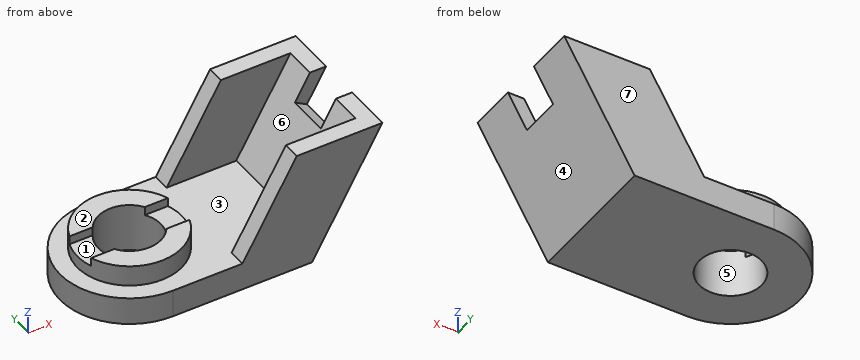
from build123d import *

# Parameters (mm, degrees)
F0_W      = 40
F0_H      = 8
F1_DEPTH  = 40
F3_DEPTH  = 8
F4_R      = 15
F5_DEPTH  = 6
F6_R      = 9
F7_DEPTH  = 14.001
F8_W      = 33.766868
F8_H      = 10
F9_DEPTH  = 2.5
F11_DEPTH = 40
F13_DEPTH = 5
F15_DEPTH = 5
F16_W     = 12
F16_H     = 11
F17_DEPTH = 5


with BuildPart() as f1:
    # F0 (on Front) → F1 (new body)
    with BuildSketch(Plane.XZ):
        with Locations((-20, -4)):
            Rectangle(F0_W, F0_H)
    extrude(amount=F1_DEPTH)

    # F2 (on face) → F3 (join)
    with BuildSketch(Plane.XY):
        with BuildLine():
            Line((-40, -40), (-40, 0))
            ThreePointArc((-40, 0), (-60, -20), (-40, -40))
        make_face()
    extrude(amount=-F3_DEPTH)

    # F4 (on face) → F5 (join)
    with BuildSketch(Plane.XY):
        with Locations((-40, -20)):
            Circle(F4_R)
    extrude(amount=F5_DEPTH)

    # F6 (on face) → F7 (cut, through all)
    with BuildSketch(Plane.XY.offset(6)):
        with Locations((-40, -20)):
            Circle(F6_R)
    extrude(amount=-F7_DEPTH, mode=Mode.SUBTRACT)

    # F8 (on face) → F9 (cut)
    with BuildSketch(Plane.XY.offset(6)):
        with Locations((-40, -20)):
            Rectangle(F8_W, F8_H)
    extrude(amount=-F9_DEPTH, mode=Mode.SUBTRACT)

    # F10 (on face) → F11 (join)
    with BuildSketch(Plane.XZ.offset(40)):
        Polygon((0, 0), (0, -8), (20.207259, 27), (15.588457, 27), align=None)
    extrude(amount=-F11_DEPTH)

    # F12 (on face) → F13 (join)
    with BuildSketch(Plane.XZ.offset(40)):
        Polygon((-4.411543, 27), (-20, 0), (0, 0), (15.588457, 27), align=None)
    extrude(amount=-F13_DEPTH)

    # F14 (on face) → F15 (join)
    with BuildSketch(Plane(origin=(0, 0, 0), x_dir=(-1, 0, 0), z_dir=(0, 1, 0))):
        Polygon((0, 0), (20, 0), (4.411543, 27), (-15.588457, 27), align=None)
    extrude(amount=-F15_DEPTH)

    # F16 (on face) → F17 (cut)
    with BuildSketch(Plane(origin=(3.464102, 0, -2), x_dir=(0, 1, 0), z_dir=(0.866025, 0, -0.5))):
        with Locations((-20, 27.986316)):
            Rectangle(F16_W, F16_H)
    extrude(amount=-F17_DEPTH, mode=Mode.SUBTRACT)


solid = f1.part
Input: part model. Units: mm. Frame: model coordinates. Face numbers are marked on the shaded views. A direction names the side the tool comes from. Coordinates: 2 decimals unless noted, no trailing zeros. Write each loop counter-clockwise with the first axis right and the second up, starting at its lowest first coordinate (ties: lowest second). Pieces come first, ordered by that corner, then holes. Notation, with made-up numbers: M -10,10.5 L 31,10.5 A8 cw 31,22.5 Z; hole C 13,38 d8. An arc over 180 degrees is marked long. Answer as a JSON object with one key per item and string values. Group by question number.
(1) Section B-B on z = 1. Output: boundary loops of the cut face in (x, y), plus the area to 3 significant figures.
(2) Ray query, line 1 along Y through (x, z) = (-40, 0.75); line 2 along Y through (x, z) = (-40, -4); line 3 along Z through (x, y) = (-54, -28). Return the intervals inside material, ascending. Write a range as [from, to].
(3) Contact query for flat-ended pins moving along their axis: P1, Ø0.8, axis at x = -28, z = 4.5, coming from the +Y side; P2, Ø3, axis at x = -11, y = -11.5, coming from the +Z side; P3, Ø16, axis at x = -40, y = -20, coming from the -Z side; P4, Ø1, axis at x = 0.5, z = -1, coming from the +Y side. Output: stop coordinate, or through.
(4) Set-up query: the marked faces 1, 2 and 3. Return all of +Z, -Z, +X, -X, +Y, -Y with unobstructed straight access to the full face (end or side cutting, diameter ignored); none if empty.
(5) Section D-D on x = -45. Output: boundary loops of the cut face in (y, z), plus the area to 3 significant figures.
(6) Section C-C on y = -8. Output: boundary loops of the cut face in (x, z).
(7) Section A-A on y = -20. Output: boundary loops of the cut face in (x, z).
(8) Mould query, pull axis Y, two halves, no side actions, for the marked faces 4, 5, 6 and 7. Classes: pulls with the +Y half, pulls with the -Y half, needs draft (parallel to the pull), parting line crosses it, or undercut.
Result set:
{
 "1": {"outline": "C -40,-20 d30; M -19.42,-40 L 5.2,-40 L 5.2,0 L -19.42,0 L -19.42,-5 L 0.58,-5 L 0.58,-35 L -19.42,-35 Z; hole C -40,-20 d18", "area": "837 mm2"},
 "2": {"line 1": "y = [-35, -29], [-11, -5]", "line 2": "y = [-40, -29], [-11, 0]", "line 3": "z = [-8, 0]"},
 "3": {"P1": "stops at y = -10.49", "P2": "stops at z = 0", "P3": "passes through", "P4": "stops at y = 0"},
 "4": {"face 1": "+Z, -X", "face 2": "+Z, -X, +Y, -Y", "face 3": "+Z"},
 "5": {"outline": "M -39.36,-8 L -27.48,-8 L -27.48,6 L -34.14,6 L -34.14,0 L -39.36,0 Z; M -12.52,-8 L -0.64,-8 L -0.64,0 L -5.86,0 L -5.86,6 L -12.52,6 Z", "area": "270 mm2"},
 "6": {"outline": "M -56,-8 L 0,-8 L 20.21,27 L 15.59,27 L 0,0 L -31,0 L -31,6 L -49,6 L -49,0 L -56,0 Z"},
 "7": {"outline": "M -60,-8 L -49,-8 L -49,3.5 L -55,3.5 L -55,0 L -60,0 Z; M -31,-8 L 0,-8 L 14.71,17.47 L 11.24,19.47 L 0,0 L -25,0 L -25,3.5 L -31,3.5 Z"},
 "8": {"face 4": "needs draft", "face 5": "undercut", "face 6": "undercut", "face 7": "pulls with the +Y half"}
}
